Read the model definition and answer for the solid it produces. Units are mm, in the model's axes. Face numbers are marked on the shaded views. A direction names the side the tool comes from. Give positions to 0.01 mm unless a question says otherwise; leave off trailing zeros. Loops run counter-clockwise (first coordinate to the right, second up) from the corner with the lowest first, then second, coordinate; pieces in that order, holes last.
(1) Find section B-B, the plane z = 3. Write down the section's boundary in (x, y) (3 decimals), then the cut area to 3 significant figures.
(2) Find section C-C, the plane x = -163.83. Write down the section's boundary in (y, z) (3 decimals).
(3) Straight lines are drawn through the part: probe 1 along X at (y, z) = (63.5, 19.5) (3 decimals); probe 2 along Z at (x, y) = (-12, 1); probe 3 along Y at (x, z) = (-24.1, 19.05). For each, find the intervals that lie inside material, in ascending order.
(4) Find section A-A, the plane x = -190.5. Write down the section's boundary in (y, z) (3 decimals), then the cut area to 3 significant figures.
(5) Which of the six approach directions +Z, -Z, +X, -X, +Y, -Y give full straight-line access (tool end or side, diameter ignored) to the marked faces 1, 2 and 3?
(6) Each of these flat-tipped pins is pushed along its axis until it touches: P1, Ø11.5, axis at y = 52.705, z = 19.05, coming from the -X side; P2, Ø4, axis at y = 57.5, z = 31.5, coming from the +X side (3 decimals); P3, Ø1.5, axis at x = -154, z = 13.5, coming from the -Y side (3 decimals); P4, Ø10, axis at y = 43.5, z = 25, coming from the -X side (3 decimals). Where does it stop, or does it pass through?
(7) Find section D-D, the plane y = 22.5. Write down the section's boundary in (x, z) (3 decimals), then the cut area to 3 significant figures.
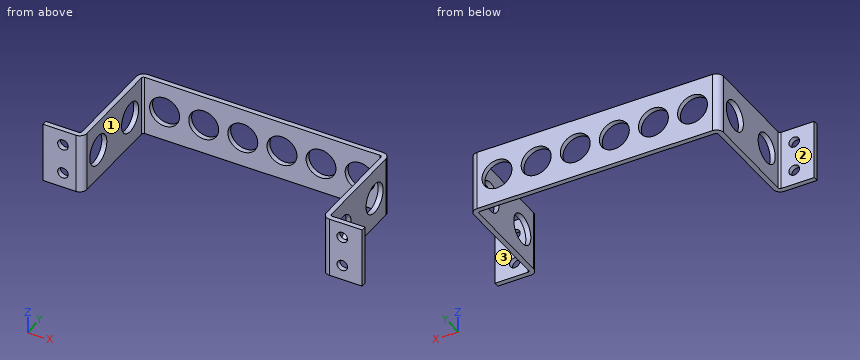
Autodesk Inventor part; units mm, degrees
ref_plane "YZ Plane" through (0, 0, 0) normal (1, 0, 0) x (0, 1, 0)
ref_plane "XZ Plane" through (0, 0, 0) normal (0, 1, 0) x (-1, 0, 0)
ref_plane "XY Plane" through (0, 0, 0) normal (0, 0, 1) x (1, 0, 0)
sketch "Sketch1" plane through (0, 0, 0) normal (0, 1, 0) x (-1, 0, 0)
  line L0 (0, 0) -> (0, 38.1)
  line L1 (0, 38.1) -> (25.4, 38.1)
  line L2 (25.4, 38.1) -> (25.4, 0)
  line L3 (25.4, 0) -> (0, 0)
  line L4 (12.7, 38.1) -> (12.7, 0) construction
  circle A0 centre (12.7, 28.575) radius 3.3782
  circle A1 centre (12.7, 9.525) radius 3.3782
  dimension "d0" = 38.1
  dimension "d1" = 25.4
  dimension "d2" = 6.7564
  dimension "d3" = 19.05
  dimension "d4" = 9.525
extrude "Plate1" add sketch "Sketch1" along normal blind 3.175
sketch "Sketch2" plane through (-22.225, 0, 38.1) normal (-1, 0, 0) x (0, -1, 0)
  line L0 (0, -38.1) -> (0, 0)
  line L1 (0, 0) -> (-69.85, 0)
  line L2 (-69.85, 0) -> (-69.85, -38.1)
  line L3 (-69.85, -38.1) -> (0, -38.1)
edge flange "Flange1" height 69.85 angle 90 thickness 3.175 bend radius 1.27 thickness toward (-1, 0, 0) relief tear relief width 3.175 relief depth 1.5875 edges at (-25.4, 3.175, 19.05) wall of the first edge with corners at (-22.225, 0, 0) (-22.225, 0, 38.1) (-22.225, 69.85, 38.1) (-22.225, 69.85, 0)
bend "Bend1"
corner "Corner1"
sketch "Sketch3" plane through (-22.225, 66.675, 0) normal (0, 1, 0) x (-1, 0, 0)
  line L0 (0, 38.1) -> (0, 0)
  line L1 (0, 0) -> (158.75, 0)
  line L2 (158.75, 0) -> (158.75, 38.1)
  line L3 (158.75, 38.1) -> (0, 38.1)
edge flange "Flange2" height 158.75 angle 90 thickness 3.175 bend radius 1.27 thickness toward (0, 1, 0) relief tear relief width 3.175 relief depth 1.5875 edges at (-25.4, 69.85, 19.05) wall of the first edge with corners at (-22.225, 66.675, 38.1) (-22.225, 66.675, 0) (-180.975, 66.675, 0) (-180.975, 66.675, 38.1)
bend "Bend2"
corner "Corner2"
sketch "Sketch4" plane through (-177.8, 69.85, 0) normal (-1, 0, 0) x (0, -1, 0)
  line L0 (0, 38.1) -> (0, 0)
  line L1 (0, 0) -> (69.85, 0)
  line L2 (69.85, 0) -> (69.85, 38.1)
  line L3 (69.85, 38.1) -> (0, 38.1)
edge flange "Flange3" height 69.85 angle 90 thickness 3.175 bend radius 1.27 thickness toward (-1, 0, 0) relief tear relief width 3.175 relief depth 1.5875 edges at (-180.975, 66.675, 19.05) wall of the first edge with corners at (-177.8, 69.85, 38.1) (-177.8, 69.85, 0) (-177.8, 0, 0) (-177.8, 0, 38.1)
bend "Bend3"
corner "Corner3"
sketch "Sketch5" plane through (-177.8, 3.175, 38.1) normal (0, -1, 0) x (1, 0, 0)
  line L0 (0, -38.1) -> (0, 0)
  line L1 (0, 0) -> (-25.4, 0)
  line L2 (-25.4, 0) -> (-25.4, -38.1)
  line L3 (-25.4, -38.1) -> (0, -38.1)
edge flange "Flange4" height 25.4 angle 90 thickness 3.175 bend radius 1.27 thickness toward (0, -1, 0) relief tear relief width 3.175 relief depth 1.5875 edges at (-180.975, 0, 19.05) wall of the first edge with corners at (-177.8, 3.175, 0) (-177.8, 3.175, 38.1) (-203.2, 3.175, 38.1) (-203.2, 3.175, 0)
bend "Bend4"
corner "Corner4"
sketch "Sketch6" plane through (-203.2, 0, 0) normal (0, -1, 0) x (1, 0, 0)
  line L0 (0, 38.1) -> (20.955, 38.1)
  line L1 (0, 0) -> (0, 38.1)
  line L2 (20.955, 0) -> (0, 0)
  line L3 (12.7, 38.1) -> (12.7, 0) construction
  circle A0 centre (12.7, 28.575) radius 3.3782
  circle A1 centre (12.7, 9.525) radius 3.3782
  point P0 (203.2, 0)
  dimension "d46" = 12.7
  dimension "d47" = 6.7564
  dimension "d48" = 19.05
  dimension "d49" = 9.525
extrude "Cut1" cut sketch "Sketch6" against normal blind 3.175
sketch "Sketch7" plane through (-26.67, 69.85, 38.1) normal (0, 1, 0) x (1, 0, 0)
  line L0 (-149.86, 38.1) -> (-149.86, 0)
  line L1 (0, 0) -> (0, 38.1)
  circle A0 centre (-137.16, 19.05) radius 9.525
  line L2 (-149.86, 19.05) -> (0, 19.05) construction
  circle A1 centre (-112.268, 19.05) radius 9.525
  circle A2 centre (-87.376, 19.05) radius 9.525
  circle A3 centre (-62.484, 19.05) radius 9.525
  circle A4 centre (-37.592, 19.05) radius 9.525
  circle A5 centre (-12.7, 19.05) radius 9.525
  point P0 (26.67, 38.1)
  dimension "d52" = 149.86
  dimension "d53" = 12.7
  dimension "d56" = 24.892
  dimension "d61" = 19.05
extrude "Cut2" cut sketch "Sketch7" against normal blind 3.175
sketch "Sketch8" plane through (-180.975, 65.405, 0) normal (-1, 0, 0) x (0, 0, 1)
  line L0 (0, -60.96) -> (38.1, -60.96)
  line L1 (38.1, 0) -> (0, 0)
  line L2 (19.05, 0) -> (19.05, -60.96) construction
  circle A0 centre (19.05, -12.7) radius 9.525
  circle A1 centre (19.05, -48.26) radius 9.525
  point P0 (0, -65.405)
  dimension "d64" = 19.05
  dimension "d66" = 12.7
  dimension "d67" = 12.7
extrude "Cut3" cut sketch "Sketch8" against normal blind 5080
equation "\"d50\" = Thickness"
equation "\"d56\" = -0.4 * d53 + 0.2 * d52"
equation "\"d62\" = Thickness"
equation "\"d6\" = BendReliefWidth"
equation "\"d7\" = BendReliefDepth"
equation "\"d8\" = MinimumRemnant"
equation "\"d9\" = BendRadius"
equation "\"d13\" = CornerReliefSize"
equation "\"d14\" = GapSize"
equation "\"d15\" = JacobiRadiusSize"
equation "\"d16\" = BendReliefWidth"
equation "\"d17\" = BendReliefDepth"
equation "\"d18\" = MinimumRemnant"
equation "\"d19\" = BendRadius"
equation "\"d23\" = CornerReliefSize"
equation "\"d24\" = GapSize"
equation "\"d25\" = JacobiRadiusSize"
equation "\"d26\" = BendReliefWidth"
equation "\"d27\" = BendReliefDepth"
equation "\"d28\" = MinimumRemnant"
equation "\"d29\" = BendRadius"
equation "\"d33\" = CornerReliefSize"
equation "\"d34\" = GapSize"
equation "\"d35\" = JacobiRadiusSize"
equation "\"d36\" = BendReliefWidth"
equation "\"d37\" = BendReliefDepth"
equation "\"d38\" = MinimumRemnant"
equation "\"d39\" = BendRadius"
equation "\"d43\" = CornerReliefSize"
equation "\"d44\" = GapSize"
equation "\"d45\" = JacobiRadiusSize"
equation "\"BendRadius\" = Thickness"
equation "\"BendReliefWidth\" = Thickness"
equation "\"BendReliefDepth\" = 0.5 * Thickness"
equation "\"CornerReliefSize\" = 4 * Thickness"
equation "\"MinimumRemnant\" = 2 * Thickness"
equation "\"TransitionRadius\" = BendRadius"
equation "\"JacobiRadiusSize\" = BendRadius"
equation "\"GapSize\" = Thickness"
equation "\"d5\" = BendRadius"
properties part number "M - Lower Rail Connector Bracket 1" material "Aluminum 6061"
Entries:
1. outline: (-203.2, 0) - (-182.245, 0) arc R4.445 ccw to (-177.8, 4.445) - (-177.8, 65.405) arc R1.27 cw to (-176.53, 66.675) - (-26.67, 66.675) arc R1.27 cw to (-25.4, 65.405) - (-25.4, 4.445) arc R4.445 ccw to (-20.955, 0) - (0, 0) - (0, 3.175) - (-20.955, 3.175) arc R1.27 cw to (-22.225, 4.445) - (-22.225, 65.405) arc R4.445 ccw to (-26.67, 69.85) - (-176.53, 69.85) arc R4.445 ccw to (-180.975, 65.405) - (-180.975, 4.445) arc R1.27 cw to (-182.245, 3.175) - (-203.2, 3.175) - close
1. area: 1,050 mm2
2. outline: (66.675, 0) - (69.85, 0) - (69.85, 9.525) - (66.675, 9.525) - close; (66.675, 28.575) - (69.85, 28.575) - (69.85, 38.1) - (66.675, 38.1) - close
3. probe 1: x = -180.975 to -177.8, -25.4 to -22.225
3. probe 2: z = 0 to 6.22, 12.83 to 25.27, 31.88 to 38.1
3. probe 3: y = 1.3 to 7.62, 26.67 to 43.18, 62.23 to 69.03
4. outline: (0, 0) - (3.175, 0) - (3.175, 6.147) - (0, 6.147) - close; (0, 12.903) - (3.175, 12.903) - (3.175, 25.197) - (0, 25.197) - close; (0, 31.953) - (3.175, 31.953) - (3.175, 38.1) - (0, 38.1) - close
4. area: 78.1 mm2
5. face 1: +Z, -Z, -Y
5. face 2: +Z, -Z, -X, +Y
5. face 3: +Z, -Z, +X, +Y
6. P1: passes through
6. P2: stops at x = -22.225
6. P3: stops at y = 66.675
6. P4: stops at x = -180.975
7. outline: (-180.975, 0) - (-177.8, 0) - (-177.8, 11.173) - (-180.975, 11.173) - close; (-180.975, 26.927) - (-177.8, 26.927) - (-177.8, 38.1) - (-180.975, 38.1) - close; (-25.4, 0) - (-22.225, 0) - (-22.225, 11.173) - (-25.4, 11.173) - close; (-25.4, 26.927) - (-22.225, 26.927) - (-22.225, 38.1) - (-25.4, 38.1) - close
7. area: 142 mm2
